Could you check a few things on this model? Use its own coordinates, in mm. A direction names the side the tool comes from. Give positions to 0.01 mm unless a question says otherwise; leave off trailing zeros. Loops run counter-clockwise (first coordinate to the right, second up) from the corner with the lowest first, then second, coordinate; pieces in that order, holes last.
1. For P1, Ø1, axis at y = 9, z = -81, coming from the -X side; P2, Ø1, axis at x = 1.5, y = -5, coming from the -Z side; P3, Ø1.5, axis at x = 2.5, y = 9, coming from the -Z side; P4, Ø4, axis at y = -11.4, z = -75.52, coming from the +X side, each with a flat end and sliding along its axis, tell me the tip position at first contact or that it passes through.
2. Thinking about a two-plate mould opening in Y: for faces 4 (the cylindrical face through (1.479, 21.874, -75.604)), 5 (the flat face through (1.479, -18.823, -87.863)), 6 (the flat face through (1.479, -25.631, -79.945)), which applies, +Y half, -Y half, draft (parallel to the pull), parting line (faces both ways), or undercut?
3. Imagine slicing it at C-C (y = 7). List the corners of the cut face in (x, z) for me.
4. Imagine slicing it at A-A (x = 1.5). List the corners of the cut face in (y, z) for me, plus the area to 3 significant figures.
5. I need wall thicknesses on line 1 along Y through (x, z) = (0.45, -89.75); line 2 along Z through (x, y) = (1, -22.5); line 3 along Y through (x, z) = (2.05, -89). Which ranges of each line are inside material? Lowest first, please.
6. For faces 1 (the flat face through (1.48, -28.61, -76.12)), 2 (the flat face through (1.48, -13.76, -89.46)), 3 (the flat face through (1.48, -24.61, -82.32)), which set-ups out of +Z, -Z, +X, -X, +Y, -Y let a thin tool reach every point of the face, with its end or its side?
7. Imagine slicing it at B-B (z = -80.25). List the corners of the cut face in (x, y) for me, plus the area to 3 significant figures.
```python
from build123d import *

# Parameters (mm, degrees)
SKETCH_1_R      = 2
SKETCH_1_R_2    = 1.5
EXTRUDE_2_DEPTH = 3


with BuildPart() as part:
    # ｽｹｯﾁ1 → ﾎﾞｽ - 押し出し2 (new body)
    with BuildSketch(Plane(origin=(0, 0, 0), x_dir=(0, 0, -1), z_dir=(1, 0, 0))):
        with BuildLine():
            ThreePointArc((79.516381724, 17.875328128), (75.516381724, 21.875328128), (71.516381724, 17.875328128))
            Line((71.516381724, 17.875328128), (71.707016231, -0.114604955))
            ThreePointArc((71.707016231, -0.114604955), (62.797189361, -13.143986116), (73.940663181, -24.323108598))
            Line((73.940663181, -24.323108598), (75.474683518, -28.648291112))
            Line((75.474683518, -28.648291112), (76.792060343, -28.56761025))
            Line((76.792060343, -28.56761025), (77.786816557, -24.087556428))
            ThreePointArc((77.786816557, -24.087556428), (78.129155766, -24.006767492), (78.469059941, -23.916279163))
            Line((78.469059941, -23.916279163), (81.461927443, -27.395239681))
            Line((81.461927443, -27.395239681), (82.661199459, -26.844115619))
            Line((82.661199459, -26.844115619), (81.970399896, -22.307242452))
            ThreePointArc((81.970399896, -22.307242452), (82.260437372, -22.108241826), (82.544700421, -21.901076422))
            Line((82.544700421, -21.901076422), (86.592211747, -24.063962049))
            Line((86.592211747, -24.063962049), (87.511410622, -23.116827145))
            Line((87.511410622, -23.116827145), (85.228351592, -19.135864493))
            ThreePointArc((85.228351592, -19.135864493), (85.426916166, -18.845528315), (85.61714679, -18.549664671))
            Line((85.61714679, -18.549664671), (90.172663107, -19.104365719))
            Line((90.172663107, -19.104365719), (90.687645941, -17.889135789))
            Line((90.687645941, -17.889135789), (87.120667215, -15.001734719))
            ThreePointArc((87.120667215, -15.001734719), (87.200941642, -14.659274498), (87.27144814, -14.314670639))
            Line((87.27144814, -14.314670639), (91.719721727, -13.186271657))
            Line((91.719721727, -13.186271657), (91.760937233, -11.867070238))
            Line((91.760937233, -11.867070238), (87.391779056, -10.463190263))
            ThreePointArc((87.391779056, -10.463190263), (84.740310623, -4.232469554), (79.205934948, -0.330822302))
            Line((79.205934948, -0.330822302), (79.516381724, 17.875328128))
        make_face()
        with Locations((75.516381724, 17.875328128)):
            Circle(SKETCH_1_R, mode=Mode.SUBTRACT)
        with Locations((75.516381724, -11.404671872)):
            Circle(SKETCH_1_R_2, mode=Mode.SUBTRACT)
    extrude(amount=EXTRUDE_2_DEPTH)


solid = part.part
```
Derived:
1. P1: passes through
1. P2: stops at z = -85.64
1. P3: stops at z = -79.38
1. P4: stops at x = 3
2. face 4: +Y half
2. face 5: undercut
2. face 6: -Y half
3. outline: (0, -79.33) - (3, -79.33) - (3, -71.63) - (0, -71.63) - close
4. outline: (-28.65, -75.47) - (-28.57, -76.79) - (-24.09, -77.79) arc R12.37 ccw to (-23.92, -78.47) - (-27.4, -81.46) - (-26.84, -82.66) - (-22.31, -81.97) arc R12.37 ccw to (-21.9, -82.54) - (-24.06, -86.59) - (-23.12, -87.51) - (-19.14, -85.23) arc R12.37 ccw to (-18.55, -85.62) - (-19.1, -90.17) - (-17.89, -90.69) - (-15, -87.12) arc R12.37 ccw to (-14.31, -87.27) - (-13.19, -91.72) - (-11.87, -91.76) - (-10.46, -87.39) arc R12.37 ccw to (-0.33, -79.21) - (17.88, -79.52) arc R4 ccw to (17.88, -71.52) - (-0.11, -71.71) arc R12.37 ccw to (-24.32, -73.94) - close; hole circle Ø3 at (-11.4, -75.52); hole circle Ø4 at (17.88, -75.52)
4. area: 679 mm2
5. line 1: y = -19.05 to -17.13, -13.69 to -11.22
5. line 2: z = -87.16 to -83.67, -82 to -68.56
5. line 3: y = -18.96 to -16.52, -13.88 to -10.98
6. face 1: -Z, +X, -X, -Y
6. face 2: -Z, +X, -X
6. face 3: +X, -X
7. outline: (0, -25.99) - (3, -25.99) - (3, -0.75) - (0, -0.75) - close
7. area: 75.7 mm2
